```python
from build123d import *

# Parameters (mm, degrees)
F0_W            = 101.6
F0_H            = 101.6
F1_DEPTH        = 914.4
F2_W            = 44.45
F2_H            = 44.45
F3_DEPTH        = 101.601
F4_W            = 44.45
F4_H            = 44.45
F5_DEPTH        = 101.601
F5_COPIES_COUNT = 3
F5_COPIES_PITCH = 508


# Not quite as in the source:
# - a pattern or mirror of a feature is missing from the dataset's text; its kind, count and spacing are read off the source's solid


with BuildPart() as f1:
    # F0 (on Right) → F1 (new body, symmetric)
    with BuildSketch(Plane.YZ):
        Rectangle(F0_W, F0_H)
    extrude(amount=F1_DEPTH, both=True)

    # F2 (on face) → F3 (cut, through all)
    with BuildSketch(Plane.XY.offset(50.8)):
        with Locations((-762, 0)):
            Rectangle(F2_W, F2_H)
    extrude(amount=-F3_DEPTH, mode=Mode.SUBTRACT)

    # F4 (on face) → F5 (cut, through all)
    with BuildSketch(Plane.XY.offset(50.8)):
        with Locations((-254, 0)):
            Rectangle(F4_W, F4_H)
    f5 = extrude(amount=-F5_DEPTH, mode=Mode.SUBTRACT)

    # F5_copies: F5 ×3
    with Locations(*[(i * F5_COPIES_PITCH, 0, 0) for i in range(1, F5_COPIES_COUNT)]):
        add(f5, mode=Mode.SUBTRACT)


solid = f1.part
```
Part model, mm, in its own coordinate system. A direction names the side the tool comes from. Give positions to 0.01 mm unless a question says otherwise; leave off trailing zeros. Write each loop counter-clockwise with the first axis right and the second up, starting at its lowest first coordinate (ties: lowest second). Pieces come first, ordered by that corner, then holes. Notation, with made-up numbers: (79.5, 0.25) -> (86.5, 0.25) arc R10 ccw to (86.5, 9.25) -> close; hole circle Ø6 at (89, 82). An arc over 180 degrees is marked (long way). Put each result on its own line as item: value. Start each with the question number.
Item 1: Cut at B-B (y = -4.5). List the corners of the cut face in (x, z) (3 decimals), then the cut area to 3 significant figures.
Item 2: Which spindle directions (+Z, -Z, +X, -X, +Y, -Y) get a long thin tool onto all of the face, cutting with end or side? Do faces 1 (the face through (-914.4, -1, 1)), 2 (the face through (254, 22.225, 1)). Say none if no direction does.
Item 3: Cut at C-C (x = 254). List the corners of the cut face in (y, z) (3 decimals).
Item 4: Pull direction Y, two halves, no side cores. Call faces 3 (the face through (13, -1, -50.8)), 4 (the face through (13, 50.8, -1)), 5 (the face through (-276.225, 0, 1)): pulls with the +Y half, pulls with the -Y half, needs draft (parallel to the pull), parting line crosses it, or undercut.
Item 5: Wall check: L1, parallel to X at y = -20.5, z = 43.5 (3 decimals); L2, parallel to Y at x = -262, z = -23.5 (3 decimals). Give the ranges that are in metal, low to high. Write a range as [from, to].
Item 6: Cut at A-A (z = -19). List the corners of the cut face in (x, y) (3 decimals), then the cut area to 3 significant figures.
Answer list:
1. outline: (-914.4, -50.8) -> (-784.225, -50.8) -> (-784.225, 50.8) -> (-914.4, 50.8) -> close; (-739.775, -50.8) -> (-276.225, -50.8) -> (-276.225, 50.8) -> (-739.775, 50.8) -> close; (-231.775, -50.8) -> (231.775, -50.8) -> (231.775, 50.8) -> (-231.775, 50.8) -> close; (276.225, -50.8) -> (739.775, -50.8) -> (739.775, 50.8) -> (276.225, 50.8) -> close; (784.225, -50.8) -> (914.4, -50.8) -> (914.4, 50.8) -> (784.225, 50.8) -> close
1. area: 168,000 mm2
2. face 1: +Z, -Z, -X, +Y, -Y
2. face 2: +Z, -Z
3. outline: (-50.8, -50.8) -> (-22.225, -50.8) -> (-22.225, 50.8) -> (-50.8, 50.8) -> close; (22.225, -50.8) -> (50.8, -50.8) -> (50.8, 50.8) -> (22.225, 50.8) -> close
4. face 3: needs draft
4. face 4: pulls with the +Y half
4. face 5: undercut
5. L1: x = [-914.4, -784.225], [-739.775, -276.225], [-231.775, 231.775], [276.225, 739.775], [784.225, 914.4]
5. L2: y = [-50.8, -22.225], [22.225, 50.8]
6. outline: (-914.4, -50.8) -> (914.4, -50.8) -> (914.4, 50.8) -> (-914.4, 50.8) -> close; hole (-784.225, -22.225) -> (-739.775, -22.225) -> (-739.775, 22.225) -> (-784.225, 22.225) -> close; hole (-276.225, -22.225) -> (-231.775, -22.225) -> (-231.775, 22.225) -> (-276.225, 22.225) -> close; hole (231.775, -22.225) -> (276.225, -22.225) -> (276.225, 22.225) -> (231.775, 22.225) -> close; hole (739.775, -22.225) -> (784.225, -22.225) -> (784.225, 22.225) -> (739.775, 22.225) -> close
6. area: 178,000 mm2
